The model under review builds one solid part; all positions refer to its coordinate system, in mm. Face numbers are marked on the shaded views. Coordinates: 2 decimals unless noted, no trailing zeros. Order: outer loops, then holes, each group sorted by start corner. A loop starts at its lowest first (then second) coordinate and runs counter-clockwise, first axis right, second up. Notation, with made-up numbers: (0, 47.25) -> (44, 47.25) arc R29 cw to (44, 80.25) -> close; hole circle Ø4 at (-39.5, 66). An arc over 180 degrees is marked (long way). Put each result on its own line as item: value.
from build123d import *

# Parameters (mm, degrees)
CUT_EXTRUDE2_REACH = 287
SKETCH3_W          = 28
SKETCH3_H          = 28
CUT_EXTRUDE3_DEPTH = 60
CUT_EXTRUDE4_REACH = 191
SKETCH7_W          = 5
SKETCH7_H          = 5
FILLET1_R          = 10


with BuildPart() as part:
    # Sketch1 → Revolve2 (revolve)
    with BuildSketch(Plane.XY):
        with BuildLine():
            Line((0, 0), (0, 40))
            Line((0, 40), (-110, 40))
            Line((-110, 40), (-110, -235))
            ThreePointArc((-110, -235), (-113.535533906, -243.535533906), (-105, -240))
            Line((-105, -240), (-105, 35))
            Line((-105, 35), (-28, 35))
            Line((-28, 35), (-28, -225))
            Line((-28, -225), (-5, -225))
            Line((-5, -225), (-5, -220))
            Line((-5, -220), (-23, -220))
            Line((-23, -220), (-23, -149))
            Line((-23, -149), (-5, -149))
            Line((-5, -149), (-5, -144))
            Line((-5, -144), (-23, -144))
            Line((-23, -144), (-23, 0))
            Line((-23, 0), (0, 0))
        make_face()
    revolve(axis=Axis((0, 0, 0), (0, 1, 0)))

    # Sketch3 → Cut-Extrude2 (cut, up to next)
    with BuildSketch(Plane(origin=(0, 40, 0), x_dir=(1, 0, 0), z_dir=(0, 1, 0)), mode=Mode.PRIVATE) as cut_extrude2_sk1:
        Rectangle(SKETCH3_W, SKETCH3_H)
    cut_extrude2_tool1 = extrude(cut_extrude2_sk1.sketch, amount=-CUT_EXTRUDE2_REACH, mode=Mode.PRIVATE) & part.part
    add(cut_extrude2_tool1.solids().sort_by_distance((0, 40, 0))[0], mode=Mode.SUBTRACT)

    # Sketch6 → Cut-Extrude3 (cut)
    with BuildSketch(Plane(origin=(0, -214.5, 0), x_dir=(1, 0, 0), z_dir=(0, 1, 0))):
        with BuildLine():
            Line((0, -28), (0, -25.5))
            ThreePointArc((0, -25.5), (3.720216095, -25.22716774), (7.360824742, -24.414509193))
            Line((7.360824742, -24.414509193), (6.639175258, -22.02092986))
            ThreePointArc((6.639175258, -22.02092986), (23, 0), (6.639175258, 22.02092986))
            Line((6.639175258, 22.02092986), (7.360824742, 24.414509193))
            ThreePointArc((7.360824742, 24.414509193), (3.720216095, 25.22716774), (0, 25.5))
            Line((0, 25.5), (0, 28))
            ThreePointArc((0, 28), (28, 0), (0, -28))
        make_face()
    extrude(amount=CUT_EXTRUDE3_DEPTH, mode=Mode.SUBTRACT)

    # Sketch7 → Cut-Extrude4 (cut, up to next)
    with BuildSketch(Plane.XZ.offset(149), mode=Mode.PRIVATE) as cut_extrude4_sk1:
        with Locations((14, 0)):
            Rectangle(SKETCH7_W, SKETCH7_H)
    cut_extrude4_tool1 = extrude(cut_extrude4_sk1.sketch, amount=-CUT_EXTRUDE4_REACH, mode=Mode.PRIVATE) & part.part
    add(cut_extrude4_tool1.solids().sort_by_distance((14, -149, 0))[0], mode=Mode.SUBTRACT)

    # Fillet1
    fillet1_edges = [part.edges().sort_by_distance(p)[0] for p in [
        (110, 40, 0),
    ]]
    fillet(fillet1_edges, radius=FILLET1_R)


solid = part.part
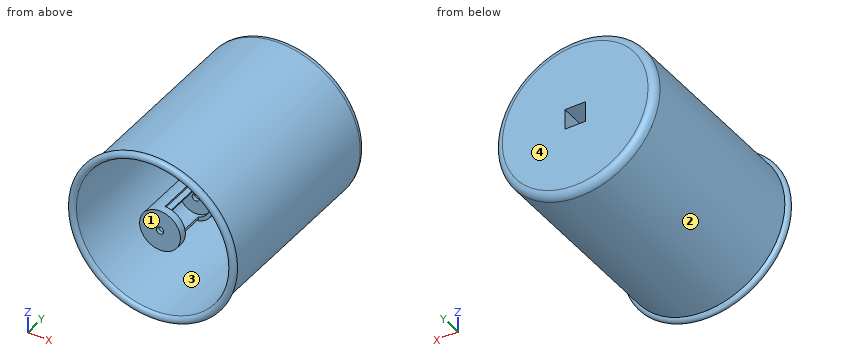
Item 1: Mouldability with a two-part tool opening along Z and no side actions: class the marked faces 1, 2, 3 and 4 as +Z half, -Z half, draft (parallel to the pull), parting line (faces both ways), or undercut.
Answers below:
face 1: undercut
face 2: parting line
face 3: undercut
face 4: draft
Item 2: Consider section A-A on y = -134. Write out the cut boundary in (x, z).
Answers below:
outline: circle Ø220 at (0, 0); circle Ø56 at (0, 0); hole circle Ø210 at (0, 0); hole circle Ø46 at (0, 0)
Item 3: For line 1 (Z direction, x = 0, y = -40.5); line 2 (Z direction, x = 17.5, y = -35.5); line 3 (Y direction, x = 19, z = -92), list the stretches that pass through material, from the lowest coordinate up. Write a range as from..to.
Answers below:
line 1: -110..-105, -28..-23, 23..28, 105..110
line 2: -108.6..-103.53, -21.86..-14.92, 14.92..21.86, 103.53..108.6
line 3: 35..40
Item 4: For pin 1 Ø6 at (x, z) = (1.5, 80.5) entering from -Y; pin 2 Ø10 at (y, z) = (-111.5, 36.5) entering from -X; pin 3 Ø2 at (x, y) = (10, -28.5) entering from -Z, all flat-tipped, find the tip position at first contact; note any pin that passes through.
Answers below:
pin 1: y = 35
pin 2: x = -105.39
pin 3: z = -109.63
